```python
from build123d import *

# Parameters (mm, degrees)
SKETCH1_W           = 50.8
SKETCH1_H           = 101.6
BOSS_EXTRUDE1_DEPTH = 5.461
SKETCH2_W           = 11.472333333
SKETCH2_H           = 5.461
SKETCH2_W_2         = 5.461
SKETCH2_H_2         = 82.55
CUT_EXTRUDE1_DEPTH  = 5.461


with BuildPart() as part:
    # Sketch1 → Boss-Extrude1 (new body)
    with BuildSketch(Plane(origin=(0, 0, 0), x_dir=(0, 0, -1), z_dir=(1, 0, 0))):
        with Locations((25.4, 50.8)):
            Rectangle(SKETCH1_W, SKETCH1_H)
    extrude(amount=BOSS_EXTRUDE1_DEPTH)

    # Sketch2 → Cut-Extrude1 (cut)
    with BuildSketch(Plane(origin=(5.461, 0, 0), x_dir=(0, 0, -1), z_dir=(1, 0, 0))):
        with Locations((45.063833333, 98.8695)):
            Rectangle(SKETCH2_W, SKETCH2_H)
        with Locations((25.4, 60.325)):
            Rectangle(SKETCH2_W_2, SKETCH2_H_2)
        with Locations((5.736166666, 98.8695)):
            Rectangle(SKETCH2_W, SKETCH2_H)
        with Locations((45.063833333, 2.7305)):
            Rectangle(SKETCH2_W, SKETCH2_H)
        with Locations((5.736166666, 2.7305)):
            Rectangle(SKETCH2_W, SKETCH2_H)
    extrude(amount=-CUT_EXTRUDE1_DEPTH, mode=Mode.SUBTRACT)


solid = part.part
```
Design review of the part built by this model. Coordinates are the model's own, in mm. A direction names the side the tool comes from. Coordinates: 2 decimals unless noted, no trailing zeros. Order: outer loops, then holes, each group sorted by start corner. A loop starts at its lowest first (then second) coordinate and runs counter-clockwise, first axis right, second up.
1) Wall thickness on line 1 along Z through (x, y) = (2.35, 59.5); line 2 along Y through (x, z) = (3.3, -11); line 3 along Y through (x, z) = (1.4, -23): over which ranges is each line inside the solid? List them lowest first.
2) Take a section at B-B, the plane x = 1.6. Give the boundary of the cut face in (y, z), and give its area (3 significant figures).
3) Take a section at C-C, the plane z = -24. Give the boundary of the cut face in (x, y), and give its area (3 significant figures).
4) For faces 1 (the flat face through (3, 3, -11.472)), 2 (the flat face through (3, 99, -11.472)), 3 (the flat face through (3, 5.461, -45)), 4 (the flat face through (3, 96.139, -45)), 5 (the flat face through (3, 60, -28.13)), list the 3-axis set-ups (+Z, -Z, +X, -X, +Y, -Y) from which the entire face can be reached by the end or side of a thin tool; tool diameter is ignored.
5) Take a section at A-A, the plane y = 44. Give the boundary of the cut face in (x, z), and give its area (3 significant figures).
6) Mouldability with a two-part tool opening along Z and no side actions: class faces 6 (the flat face through (3, 99, -39.328)), 7 (the flat face through (3, 19.05, -25)), 8 (the flat face through (3, 101.6, -17)) as +Z half, -Z half, draft (parallel to the pull), parting line (faces both ways), or undercut.
7) Take a section at D-D, the plane z = -9. Give the boundary of the cut face in (x, y).
8) Clearance check with flat-ended pins moving along their axes: pin 1 (1.6 mm diameter, centred on x = 2, z = -6.5, fed in from -Y); pin 2 (2.5 mm diameter, centred on x = 2, y = 99, fed in from +Z); pin 3 (2.5 mm diameter, centred on x = 4, y = 100, fed in from -Z). State where each tip first meets the part, or that it passes through.
Returned:
1. line 1: z = -50.8 to -28.13, -22.67 to 0
1. line 2: y = 5.46 to 96.14
1. line 3: y = 0 to 19.05
2. outline: (0, -39.33) - (5.46, -39.33) - (5.46, -50.8) - (96.14, -50.8) - (96.14, -39.33) - (101.6, -39.33) - (101.6, -28.13) - (19.05, -28.13) - (19.05, -22.67) - (101.6, -22.67) - (101.6, -11.47) - (96.14, -11.47) - (96.14, 0) - (5.46, 0) - (5.46, -11.47) - (0, -11.47) - close
2. area: 4,460 mm2
3. outline: (0, 0) - (5.46, 0) - (5.46, 19.05) - (0, 19.05) - close
3. area: 104 mm2
4. face 1: +Z, +X, -X, -Y
4. face 2: +Z, +X, -X, +Y
4. face 3: -Z, +X, -X, -Y
4. face 4: -Z, +X, -X, +Y
4. face 5: +X, -X, +Y
5. outline: (0, -50.8) - (5.46, -50.8) - (5.46, -28.13) - (0, -28.13) - close; (0, -22.67) - (5.46, -22.67) - (5.46, 0) - (0, 0) - close
5. area: 248 mm2
6. face 6: -Z half
6. face 7: undercut
6. face 8: draft
7. outline: (0, 5.46) - (5.46, 5.46) - (5.46, 96.14) - (0, 96.14) - close
8. pin 1: stops at y = 5.46
8. pin 2: stops at z = -11.47
8. pin 3: stops at z = -39.33
